For this review, take the finished solid that the model builds, in its own axes (mm). A direction names the side the tool comes from. Round coordinates to 2 decimals unless told otherwise and drop trailing zeros. One line per item, written item: value.
```python
from build123d import *

# Parameters (mm, degrees)
SKETCH1_R                = 29.0703
BOSS_EXTRUDE2_DEPTH      = 4.7625
FILLET1_R                = 3.175
SKETCH2_W                = 14.732
SKETCH2_H                = 10.414
CUT_EXTRUDE2_DEPTH       = 12.7
CIRPATTERN1_COUNT        = 7
SKETCH4_R                = 1.143
CUT_EXTRUDE4_DEPTH       = 9.525
CIRPATTERN2_COUNT        = 7
SKETCH5_W                = 6.477
SKETCH5_H                = 6.477
CUT_EXTRUDE5_DEPTH       = 42.376236281
SKETCH6_R                = 2.286
CUT_EXTRUDE7_DEPTH       = 42.376236281
SKETCH7_R                = 4.445
CUT_EXTRUDE8_DEPTH       = 2.54
BOSS_EXTRUDE4_REACH      = 48.843
FILLET2_R                = 0.127
CIRPATTERN5_COUNT        = 7
FILLET2_OF_CIRPATTERN5_R = 0.127
FILLET3_R                = 1.016


with BuildPart() as part:
    # Sketch1 → Boss-Extrude2 (new body)
    with BuildSketch(Plane.XY):
        Circle(SKETCH1_R)
    extrude(amount=-BOSS_EXTRUDE2_DEPTH)

    # Fillet1
    fillet1_edges = [part.edges().sort_by_distance(p)[0] for p in [
        (-29.0703, 0, -4.7625),
    ]]
    fillet(fillet1_edges, radius=FILLET1_R)

    # Sketch2 → Cut-Extrude2 (cut)
    with BuildSketch(Plane.XY):
        with Locations((0, 25.1333)):
            Rectangle(SKETCH2_W, SKETCH2_H)
    cut_extrude2 = extrude(amount=-CUT_EXTRUDE2_DEPTH, mode=Mode.SUBTRACT)

    # CirPattern1: Cut-Extrude2 ×7 about axis
    cirpattern1_axis = Axis((0, 0, 0), (0, 0, 1))
    for i in range(1, CIRPATTERN1_COUNT):
        add(cut_extrude2.rotate(cirpattern1_axis, i * 360 / CIRPATTERN1_COUNT), mode=Mode.SUBTRACT)

    # Sketch4 → Cut-Extrude4 (cut, symmetric)
    with BuildSketch(Plane(origin=(0, 0, 0), x_dir=(0, 0, -1), z_dir=(1, 0, 0))):
        with Locations((0, 25.7683)):
            Circle(SKETCH4_R)
    cut_extrude4 = extrude(amount=CUT_EXTRUDE4_DEPTH, both=True, mode=Mode.SUBTRACT)

    # CirPattern2: Cut-Extrude4 ×7 about axis
    cirpattern2_axis = Axis((0, 0, 0), (0, 0, 1))
    for i in range(1, CIRPATTERN2_COUNT):
        add(cut_extrude4.rotate(cirpattern2_axis, i * 360 / CIRPATTERN2_COUNT), mode=Mode.SUBTRACT)

    # Sketch5 → Cut-Extrude5 (cut, through all)
    with BuildSketch(Plane.XY):
        Rectangle(SKETCH5_W, SKETCH5_H)
    extrude(amount=-CUT_EXTRUDE5_DEPTH, mode=Mode.SUBTRACT)

    # Sketch6 → Cut-Extrude7 (cut, through all)
    with BuildSketch(Plane(origin=(0, 0, -4.7625), x_dir=(-1, 0, 0), z_dir=(0, 0, -1))):
        with Locations((12.7, 0)):
            Circle(SKETCH6_R)
        with Locations((0, -12.7)):
            Circle(SKETCH6_R)
        with Locations((-12.7, 0)):
            Circle(SKETCH6_R)
        with Locations((0, 12.7)):
            Circle(SKETCH6_R)
    extrude(amount=-CUT_EXTRUDE7_DEPTH, mode=Mode.SUBTRACT)

    # Sketch7 → Cut-Extrude8 (cut)
    with BuildSketch(Plane(origin=(0, 0, -4.7625), x_dir=(-1, 0, 0), z_dir=(0, 0, -1))):
        with Locations((12.7, 0)):
            Circle(SKETCH7_R)
        with Locations((0, -12.7)):
            Circle(SKETCH7_R)
        with Locations((-12.7, 0)):
            Circle(SKETCH7_R)
        with Locations((0, 12.7)):
            Circle(SKETCH7_R)
    extrude(amount=-CUT_EXTRUDE8_DEPTH, mode=Mode.SUBTRACT)

    # Sketch10 → Boss-Extrude4 (add, up to next)
    with BuildSketch(Plane.ZY.offset(-7.366), mode=Mode.PRIVATE) as boss_extrude4_sk1:
        with BuildLine():
            Line((-4.7625, 19.9263), (0, 19.9263))
            Line((0, 19.9263), (0, 20.0533))
            ThreePointArc((0, 20.0533), (-2.7025038, 20.73265722), (-4.7625, 22.609214887))
            Line((-4.7625, 22.609214887), (-4.7625, 19.9263))
        make_face()
    boss_extrude4_tool1 = extrude(boss_extrude4_sk1.sketch, amount=BOSS_EXTRUDE4_REACH, mode=Mode.PRIVATE) - part.part
    boss_extrude4 = boss_extrude4_tool1.solids().sort_by_distance((7.366, 20.664807, -3.452063))[0]
    add(boss_extrude4)

    # Fillet2
    fillet2_edges = [part.edges().sort_by_distance(p)[0] for p in [
        (0, 22.609214887, -4.7625),
    ]]
    fillet(fillet2_edges, radius=FILLET2_R)

    # CirPattern5: Boss-Extrude4 ×7 about axis
    cirpattern5_axis = Axis((0, 0, 0), (0, 0, 1))
    for i in range(1, CIRPATTERN5_COUNT):
        add(boss_extrude4.rotate(cirpattern5_axis, i * 360 / CIRPATTERN5_COUNT))

    # Fillet2 of CirPattern5
    fillet2_of_cirpattern5_edges = [part.edges().sort_by_distance(p)[0] for p in [
        (-17.676595993, 14.09661491, -4.7625),
        (-22.042354666, -5.031023613, -4.7625),
        (-9.809770694, -20.370198741, -4.7625),
        (9.809770694, -20.370198741, -4.7625),
        (22.042354666, -5.031023613, -4.7625),
        (17.676595993, 14.09661491, -4.7625),
    ]]
    fillet(fillet2_of_cirpattern5_edges, radius=FILLET2_OF_CIRPATTERN5_R)

    # Fillet3
    fillet3_edges = [part.edges().sort_by_distance(p)[0] for p in [
        (3.2385, 3.2385, -2.38125),
        (3.2385, -3.2385, -2.38125),
        (-3.2385, -3.2385, -2.38125),
        (-3.2385, 3.2385, -2.38125),
    ]]
    fillet(fillet3_edges, radius=FILLET3_R)


solid = part.part
```
Item 1: Take a section at A-A (x = 0). Count the separate pieces of the cut face and the enclosed holes in it, plus the area to 3 significant figures.
Returned:
separate pieces: 4
enclosed holes: 0
area: 139 mm^2
Item 2: Wall thickness on line 1 (Y direction, x = 0, z = -1.7); line 2 (X direction, y = 11, z = -1.9); line 3 (Y direction, x = 12.7, z = -2.85) (3 decimals): over which ranges is each line inside the solid? List them lowest first.
Returned:
line 1: -29.07 to -14.99, -10.41 to -3.24, 3.24 to 10.41, 14.99 to 20.31
line 2: -26.89 to -25.61, -17.29 to -1.53, 1.53 to 17.29, 25.61 to 26.89
line 3: -16.987 to -4.445, 4.445 to 17.459, 19.549 to 25.858
Item 3: For P1, Ø3.5, axis at x = 0, y = -12.7, coming from the -Z side; P2, Ø1, axis at x = -8.5, z = -2.5, coming from the +Y side; P3, Ø2, axis at y = -0.5, z = -1, coming from the -X side; P4, Ø1.3, axis at y = -1, z = -3.5, coming from the +X side, all flat-tipped, find the tip position at first contact; note any pin that passes through.
Returned:
P1: through
P2: y = 27.86
P3: x = -20.89
P4: x = 22.19
Item 4: The part is to be moulded in two halves that separate along X. For faces 1 (the flat face through (5, 3, 0)), 2 (the cylindrical face through (13, 26, -1)), 3 (the cylindrical face through (14.871, 22.642, -1.143)), say which applies: +X half, -X half, draft (parallel to the pull), parting line (faces both ways), or undercut.
Returned:
face 1: draft
face 2: +X half
face 3: undercut
Item 5: Machinability: for faces 4 (the flat face through (21.79, -12.53, -2.35)), 5 (the cylindrical face through (0.96, 8.36, -3.51)), 6 (the cylindrical face through (0.5, -14.93, -1.13)), 7 (the flat face through (26.1, 8.63, -0.44)), 8 (the cylindrical face through (28.36, 6.39, -0.78)), which of the approach directions +Z, -Z, +X, -X, +Y, -Y give a long, thin tool a straight path to every point of the face, cutting with its end or side? Answer none if there is none.
Returned:
face 4: +Z, +X
face 5: -Z
face 6: +Z, -Z
face 7: +Z
face 8: +Z, -Z, +X, +Y
